Verification items for the finished model (mm, model axes). Face numbers are marked on the shaded views. A direction names the side the tool comes from. Coordinates: 2 decimals unless noted, no trailing zeros. Order: outer loops, then holes, each group sorted by start corner. A loop starts at its lowest first (then second) coordinate and runs counter-clockwise, first axis right, second up. Notation, with made-up numbers: M 86,31.5 L 101,31.5 A34 ccw 101,64.5 Z; hole C -19,-5.5 d3. An arc over 180 degrees is marked long. Return JSON: item names as keys, results as strings.
```python
from build123d import *

# Parameters (mm, degrees)
BOX001_W     = 20
BOX001_H     = 20
BOX001_DEPTH = 101
BOX002_W     = 20
BOX002_H     = 20
BOX002_DEPTH = 101
BOX003_W     = 20
BOX003_H     = 20
BOX003_DEPTH = 101
BOX004_W     = 20
BOX004_H     = 20
BOX004_DEPTH = 101
BOX_W        = 200
BOX_H        = 200
BOX_DEPTH    = 5


with BuildPart() as obj1:
    # Box001 → Box001 (new body)
    with BuildSketch(Plane(origin=(10, 10, -100), x_dir=(1, 0, 0), z_dir=(0, 0, 1))):
        with Locations((10, 10)):
            Rectangle(BOX001_W, BOX001_H)
    extrude(amount=BOX001_DEPTH)


with BuildPart() as box002:
    # Box002 → Box002 (new body)
    with BuildSketch(Plane(origin=(170, 10, -100), x_dir=(1, 0, 0), z_dir=(0, 0, 1))):
        with Locations((10, 10)):
            Rectangle(BOX002_W, BOX002_H)
    extrude(amount=BOX002_DEPTH)


with BuildPart() as box003:
    # Box003 → Box003 (new body)
    with BuildSketch(Plane(origin=(10, 170, -100), x_dir=(1, 0, 0), z_dir=(0, 0, 1))):
        with Locations((10, 10)):
            Rectangle(BOX003_W, BOX003_H)
    extrude(amount=BOX003_DEPTH)


with BuildPart() as box004:
    # Box004 → Box004 (new body)
    with BuildSketch(Plane(origin=(170, 170, -100), x_dir=(1, 0, 0), z_dir=(0, 0, 1))):
        with Locations((10, 10)):
            Rectangle(BOX004_W, BOX004_H)
    extrude(amount=BOX004_DEPTH)


with BuildPart() as mesa:
    # Box → Box (new body)
    with BuildSketch(Plane.XY):
        with Locations((100, 100)):
            Rectangle(BOX_W, BOX_H)
    extrude(amount=BOX_DEPTH)

    # Fusion: union obj1, Box002, Box003, Box004
    add(obj1.part)
    add(box002.part)
    add(box003.part)
    add(box004.part)


solid = mesa.part
```
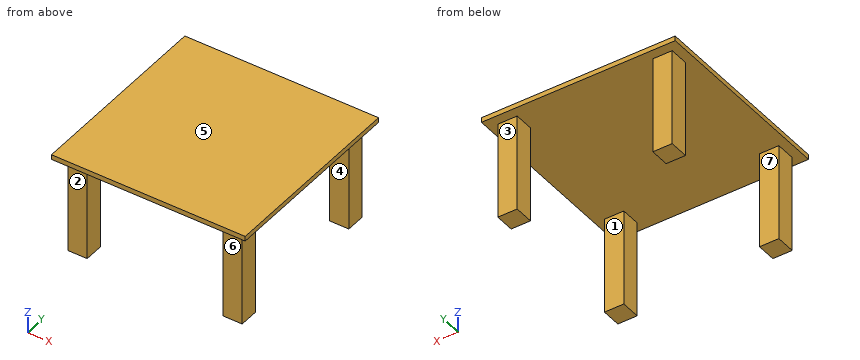
Q1. Go/stop test with flat-tipped pins: pin 1 (22 mm diameter, centred on x = 182.5, z = -73.5, fed in from -Y); pin 2 (22 mm diameter, centred on y = 180.5, z = -60, fed in from -X); pin 3 (10 mm diameter, centred on x = 32.5, y = 92, fed in from -Z). Record where each tip stops, or that it passes through.
Values:
{"pin 1": "y = 10", "pin 2": "x = 10", "pin 3": "z = 0"}
Q2. Draft check along Y on the marked faces 4, 5, 6 and 7. Enter one of: pulls with the +Y half, pulls with the -Y half, needs draft (parallel to the pull), parting line crosses it, or undercut.
Values:
{"face 4": "undercut", "face 5": "needs draft", "face 6": "pulls with the -Y half", "face 7": "undercut"}
Q3. Tool access check on the marked faces 1, 2 and 3. Record the directions out of +Z, -Z, +X, -X, +Y, -Y that give a thin tool (end or side, any length) a straight path to the whole face; none if there is none.
Values:
{"face 1": "-Z, +X, -X", "face 2": "-Z, +X, -X, -Y", "face 3": "-Z, +X, -X, +Y"}
Q4. Cross-section at B-B, the plane x = 17.5. Record the boundary of the cut face in (y, z), and give its area (3 significant figures).
Values:
{"outline": "M 0,0 L 10,0 L 10,-100 L 30,-100 L 30,0 L 170,0 L 170,-100 L 190,-100 L 190,0 L 200,0 L 200,5 L 0,5 Z", "area": "5,000 mm^2"}
Q5. Cross-section at D-D, the plane x = 57.5. Record the boundary of the cut face in (y, z), and give its area (3 significant figures).
Values:
{"outline": "M 0,0 L 200,0 L 200,5 L 0,5 Z", "area": "1,000 mm^2"}
Q6. Cross-section at A-A, the plane z = -40. Record the boundary of the cut face in (x, y), and give its area (3 significant figures).
Values:
{"outline": "M 10,10 L 30,10 L 30,30 L 10,30 Z; M 10,170 L 30,170 L 30,190 L 10,190 Z; M 170,10 L 190,10 L 190,30 L 170,30 Z; M 170,170 L 190,170 L 190,190 L 170,190 Z", "area": "1,600 mm^2"}
Q7. Material ranges on line 1 along Y through (x, z) = (16, -42.5); line 2 along Z through (x, y) = (48, 64.5), recorded low to high.
Values:
{"line 1": "10 to 30, 170 to 190", "line 2": "0 to 5"}
